Source: CAD feature listing. Evaluate the final solid. Frame: model axes, mm. A direction names the side the tool comes from. Coordinates: 2 decimals unless noted, no trailing zeros. Order: outer loops, then holes, each group sorted by start corner. A loop starts at its lowest first (then second) coordinate and runs counter-clockwise, first axis right, second up.
Item 1: Contact query for flat-ended pins moving along their axis: P1, Ø4.5, axis at x = 11.525, y = 5.025, coming from the -Z side; P2, Ø3, axis at y = 3, z = -3, coming from the -X side. Output: stop coordinate, or through.
Item 2: Mould query, pull axis Y, two halves, no side actions, for faces 1 (the cylindrical face through (10.174, 5.084, -3.131)), 2 (the flat face through (3, 9.525, -5)), 3 (the flat face through (21, 0, -3)). Classes: released by +Y, released by -Y, zero draft, split by the parting line, or undercut.
Item 3: Section A-A on x = -12. Return the cut outline in (y, z) (3 decimals).
Item 4: Reachability of faces 4 (the cylindrical face through (11.232, -6.345, -3.131)), 5 (the flat face through (-18, -1.143, -3)) from +Z, -Z, +X, -X, +Y, -Y: full face, straight path, thin tool, end or side. Return the list, or none.
Item 5: Section C-C on x = -5. Return the cut outline in (y, z) (3 decimals).
Item 6: Ray query, line 1 (X direction, y = -5, z = -3.75); line 2 (X direction, y = -8, z = -1.5); line 3 (Y direction, x = 10.5, z = -5) (3 decimals). Return the intervals inside material, ascending.
Item 7: Section B-B on y = 1.5. Return the cut outline in (x, z) (3 decimals).
Item 8: Section D-D on z = -5.5. Return the cut outline in (x, y) (3 decimals), then the cut area to 3 significant figures.
from build123d import *

# Parameters (mm, degrees)
BOSS_EXTRUDE1_DEPTH       = 21
F_6_32_TAPPED_HOLE1_D     = 2.7051
F_6_32_TAPPED_HOLE1_DEPTH = 9.398
F_6_32_TAPPED_HOLE1_TIP   = 0.81269403
F_6_CLEARANCE_HOLE1_D     = 3.6576
FILLET1_R                 = 0.75
SKETCH8_W                 = 6
SKETCH8_H                 = 10.668
CUT_EXTRUDE1_DEPTH        = 24.917527635


with BuildPart() as part:
    # Sketch1 → Boss-Extrude1 (new, symmetric)
    with BuildSketch(Plane(origin=(0, 0, 0), x_dir=(0, 0, -1), z_dir=(1, 0, 0))):
        Polygon((0, 6.35), (3.175, 9.525), (6.35, 9.525), (6.35, -9.525), (0, -9.525), align=None)
    extrude(amount=BOSS_EXTRUDE1_DEPTH, both=True)

    # #6-32 Tapped Hole1
    with Locations(Plane(origin=(0, 0, -6.35), x_dir=(-1, 0, 0), z_dir=(0, 0, -1))):
        with Locations((11.525, -5.025), (-11.525, 5.025), (-11.525, -5.025), (11.525, 5.025)):
            Hole(F_6_32_TAPPED_HOLE1_D / 2, depth=F_6_32_TAPPED_HOLE1_DEPTH)
            with Locations((0, 0, -(F_6_32_TAPPED_HOLE1_DEPTH + F_6_32_TAPPED_HOLE1_TIP / 2))):  # 118° drill point
                Cone(0, F_6_32_TAPPED_HOLE1_D / 2, F_6_32_TAPPED_HOLE1_TIP, mode=Mode.SUBTRACT)

    # #6 Clearance Hole1 (through all)
    with Locations(Plane(origin=(0, -9.525, 0), x_dir=(-1, 0, 0), z_dir=(0, -1, 0))):
        with Locations((-15.525, 0), (15.525, 0)):
            Hole(F_6_CLEARANCE_HOLE1_D / 2)

    # Fillet1
    # the kernel refuses this fillet: 0.75 mm, written as the material it takes off along each edge
    with BuildSketch(Plane(origin=(-14.472850429, 6.35, 0), x_dir=(0, 0.707106781186552, -0.7071067811865431), z_dir=(1, 0, 0)), Plane(origin=(11.019949465, 6.35, 0), x_dir=(0, 0.707106781186552, -0.7071067811865431), z_dir=(1, 0, 0))) as fillet1_piece_1:
        with BuildLine():
            CenterArc((FILLET1_R * 0.414213562373, -FILLET1_R), FILLET1_R, 90, 45)
            Line((-FILLET1_R * 0.292893218813, -FILLET1_R * 0.292893218813), (0, 0))
            Line((0, 0), (FILLET1_R * 0.414213562373, 0))
        make_face()
    extrude(amount=3.452900965, mode=Mode.SUBTRACT)
    with BuildSketch(Plane(origin=(-12.030050535, 6.35, 0), x_dir=(0, 0.707106781186552, -0.7071067811865431), z_dir=(1, 0, 0))) as fillet1_piece_2:
        with BuildLine():
            CenterArc((FILLET1_R * 0.414213562373, -FILLET1_R), FILLET1_R, 90, 45)
            Line((-FILLET1_R * 0.292893218813, -FILLET1_R * 0.292893218813), (0, 0))
            Line((0, 0), (FILLET1_R * 0.414213562373, 0))
        make_face()
    extrude(amount=24.060101071, mode=Mode.SUBTRACT)
    with BuildSketch(Plane(origin=(-15.5712, -9.525, 0), x_dir=(0, 1, 0), z_dir=(1, 0, 0))) as fillet1_piece_3:
        with BuildLine():
            CenterArc((FILLET1_R, -FILLET1_R), FILLET1_R, 90, 90)
            Line((0, -FILLET1_R), (0, 0))
            Line((0, 0), (FILLET1_R, 0))
        make_face()
    extrude(amount=31.1424, mode=Mode.SUBTRACT)

    # Sketch8 → Cut-Extrude1 (cut, through all)
    with BuildSketch(Plane.XY):
        with Locations((-18, 4.191)):
            Rectangle(SKETCH8_W, SKETCH8_H)
    extrude(amount=-CUT_EXTRUDE1_DEPTH, mode=Mode.SUBTRACT)


solid = part.part
Answer list:
1. P1: stops at z = -6.35
1. P2: stops at x = -15
2. face 1: undercut
2. face 2: released by +Y
2. face 3: zero draft
3. outline: (-9.525, -6.35) - (-6.291, -6.35) - (-6.291, 0) - (-8.775, 0) arc R0.75 ccw to (-9.525, -0.75) - close; (-3.759, -6.35) - (3.759, -6.35) - (3.759, 0) - (-3.759, 0) - close; (6.291, -6.35) - (9.525, -6.35) - (9.525, -3.175) - (6.57, -0.22) arc R0.75 ccw to (6.291, -0.044) - close
4. face 4: +Z, -Z
4. face 5: +Z, -Z, -X, +Y
5. outline: (-9.525, -6.35) - (9.525, -6.35) - (9.525, -3.175) - (6.57, -0.22) arc R0.75 ccw to (6.039, 0) - (-8.775, 0) arc R0.75 ccw to (-9.525, -0.75) - close
6. line 1: x = -21 to -12.88, -10.17 to 10.17, 12.88 to 21
6. line 2: x = -21 to -16.57, -14.48 to 14.48, 16.57 to 21
6. line 3: y = -9.525 to -5.907, -4.143 to 4.143, 5.907 to 9.525
7. outline: (-15, -6.35) - (21, -6.35) - (21, 0) - (17.354, 0) arc R1.829 cw to (13.696, 0) - (-13.696, 0) arc R1.829 cw to (-15, -1.752) - close
8. outline: (-21, -9.525) - (21, -9.525) - (21, 9.525) - (-15, 9.525) - (-15, -1.143) - (-21, -1.143) - close; hole circle Ø2.705 at (-11.525, -5.025); hole circle Ø2.705 at (-11.525, 5.025); hole circle Ø2.705 at (11.525, -5.025); hole circle Ø2.705 at (11.525, 5.025)
8. area: 713 mm2
